Part model, mm, in its own coordinate system. Face numbers are marked on the shaded views. A direction names the side the tool comes from. Give positions to 0.01 mm unless a question says otherwise; leave off trailing zeros. Order: outer loops, then holes, each group sorted by start corner. A loop starts at its lowest first (then second) coordinate and runs counter-clockwise, first axis right, second up.
from build123d import *

# Parameters (mm, degrees)
SKETCH1_R                    = 37.5
BOSS_EXTRUDE1_DEPTH          = 6
CSK_FOR_M3_SFHCS1_AT_2_COUNT = 2
CSK_FOR_M3_SFHCS1_AT_2_PITCH = 17.32
CSK_FOR_M3_SFHCS1_AT_3_COUNT = 2
CSK_FOR_M3_SFHCS1_AT_3_PITCH = 17.32
SKETCH5_OUTSIDE_W            = 98.248
SKETCH5_OUTSIDE_H            = 98.248
SKETCH5_OUTSIDE_R            = 31
CUT_EXTRUDE2_DEPTH           = 3
F_4_0MM_DOWEL_HOLE1_D        = 4.2
F_4_0MM_DOWEL_HOLE1_DEPTH    = 10
F_4_0MM_DOWEL_HOLE1_TIP      = 1.2618073
CUT_EXTRUDE3_DEPTH           = 3.3
CHAMFER1_SIZE                = 0.5


with BuildPart() as part:
    # Sketch1 → Boss-Extrude1 (new body)
    with BuildSketch(Plane(origin=(0, 0, 0), x_dir=(1, 0, 0), z_dir=(0, 1, 0))):
        with Locations(Location((0, 0, 0), (0, 0, 270))):
            Circle(SKETCH1_R)
    extrude(amount=BOSS_EXTRUDE1_DEPTH)

    # Sketch3 → CSK for M3 SFHCS1 (revolve, cut)
    with BuildSketch(Plane(origin=(8.66, 6, 4.999853331), x_dir=(0, 0, 1), z_dir=(1, 0, 0))):
        Polygon((0, 0), (0, 11.021463052), (1.7, 10), (1.7, 2.66), (3.36, 1), (3.36, 0), align=None)
    csk_for_m3_sfhcs1 = revolve(axis=Axis((8.66, 12.35, 4.999853331), (0, -1, 0)), mode=Mode.SUBTRACT)

    # CSK for M3 SFHCS1 at 2: CSK for M3 SFHCS1 ×2
    with Locations(*[Vector(-0.5000000000000001, 0, -0.8660254037844387) * (i * CSK_FOR_M3_SFHCS1_AT_2_PITCH) for i in range(1, CSK_FOR_M3_SFHCS1_AT_2_COUNT)]):
        add(csk_for_m3_sfhcs1, mode=Mode.SUBTRACT)

    # CSK for M3 SFHCS1 at 3: CSK for M3 SFHCS1 ×2
    with Locations(*[(-i * CSK_FOR_M3_SFHCS1_AT_3_PITCH, 0, 0) for i in range(1, CSK_FOR_M3_SFHCS1_AT_3_COUNT)]):
        add(csk_for_m3_sfhcs1, mode=Mode.SUBTRACT)

    # Sketch5 outside → Cut-Extrude2 (cut)
    with BuildSketch(Plane(origin=(0, 6, 0), x_dir=(1, 0, 0), z_dir=(0, 1, 0))):
        Rectangle(SKETCH5_OUTSIDE_W, SKETCH5_OUTSIDE_H)
        with Locations(Location((0, 0, 0), (0, 0, 270))):
            Circle(SKETCH5_OUTSIDE_R, mode=Mode.SUBTRACT)
    extrude(amount=-CUT_EXTRUDE2_DEPTH, mode=Mode.SUBTRACT)

    # Ø4.0mm Dowel Hole1
    with Locations(Plane(origin=(0, 6, 0), x_dir=(1, 0, 0), z_dir=(0, 1, 0))):
        with Locations((17.67766953, 17.67766953), (-17.67766953, 17.67766953), (17.67766953, -17.67766953), (-17.67766953, -17.67766953)):
            Hole(F_4_0MM_DOWEL_HOLE1_D / 2, depth=F_4_0MM_DOWEL_HOLE1_DEPTH)
            with Locations((0, 0, -(F_4_0MM_DOWEL_HOLE1_DEPTH + F_4_0MM_DOWEL_HOLE1_TIP / 2))):  # 118° drill point
                Cone(0, F_4_0MM_DOWEL_HOLE1_D / 2, F_4_0MM_DOWEL_HOLE1_TIP, mode=Mode.SUBTRACT)

    # Sketch8 → Cut-Extrude3 (cut)
    with BuildSketch(Plane.XZ):
        Polygon((-14.22766953, 15.685811101), (-14.22766953, 19.669527958), (-17.67766953, 21.661386387), (-21.12766953, 19.669527958), (-21.12766953, 15.685811101), (-17.67766953, 13.693952672), align=None)
        Polygon((17.67766953, 13.693952672), (21.12766953, 15.685811101), (21.12766953, 19.669527958), (17.67766953, 21.661386387), (14.22766953, 19.669527958), (14.22766953, 15.685811101), align=None)
        Polygon((14.22766953, -19.669527958), (17.67766953, -21.661386387), (21.12766953, -19.669527958), (21.12766953, -15.685811101), (17.67766953, -13.693952672), (14.22766953, -15.685811101), align=None)
        Polygon((-14.22766953, -19.669527958), (-14.22766953, -15.685811101), (-17.67766953, -13.693952672), (-21.12766953, -15.685811101), (-21.12766953, -19.669527958), (-17.67766953, -21.661386387), align=None)
    extrude(amount=-CUT_EXTRUDE3_DEPTH, mode=Mode.SUBTRACT)

    # Chamfer1
    chamfer1_edges = [part.edges().sort_by_distance(p)[0] for p in [
        (15.95266953, 0, 14.689881887),
        (19.40266953, 0, 14.689881887),
        (21.12766953, 0, 17.67766953),
        (19.40266953, 0, 20.665457173),
        (15.95266953, 0, 20.665457173),
        (14.22766953, 0, 17.67766953),
        (-15.95266953, 0, 14.689881887),
        (-14.22766953, 0, 17.67766953),
        (-15.95266953, 0, 20.665457173),
        (-19.40266953, 0, 20.665457173),
        (-21.12766953, 0, 17.67766953),
        (-19.40266953, 0, 14.689881887),
        (-8.66, 0, 3.299853331),
        (-8.66, 6, 1.639853331),
        (0, 0, -37.5),
        (0, 0, -11.699706662),
        (0, 6, -13.359706662),
        (0, 3, -37.5),
        (0, 6, -31),
        (19.77766953, 6, -17.67766953),
        (-15.57766953, 6, 17.67766953),
        (19.77766953, 6, 17.67766953),
        (-15.57766953, 6, -17.67766953),
        (8.66, 0, 3.299853331),
        (8.66, 6, 1.639853331),
        (-15.95266953, 0, -20.665457173),
        (-14.22766953, 0, -17.67766953),
        (-15.95266953, 0, -14.689881887),
        (-19.40266953, 0, -14.689881887),
        (-21.12766953, 0, -17.67766953),
        (-19.40266953, 0, -20.665457173),
        (14.22766953, 0, -17.67766953),
        (15.95266953, 0, -20.665457173),
        (19.40266953, 0, -20.665457173),
        (21.12766953, 0, -17.67766953),
        (19.40266953, 0, -14.689881887),
        (15.95266953, 0, -14.689881887),
    ]]
    chamfer(chamfer1_edges, length=CHAMFER1_SIZE)


solid = part.part
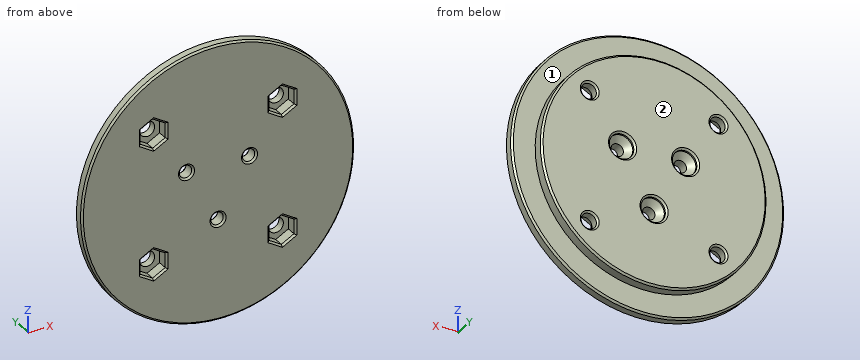
Item 1: Band-saw the part on A-A on x = 0. List the corners of the cut face in (y, z).
Item 2: Band-saw the part on B-B on z = 0. List the corners of the cut face in (x, y).
Item 3: Which spindle directions (+Z, -Z, +X, -X, +Y, -Y) get a long thin tool onto all of the face, cutting with end or side? Do the marked faces 1 and 2. Say none if no direction does.
Item 4: Drill centre lines: probe 1 along X at (y, z) = (5, 5); probe 2 along Z at (x, y) = (0, 2.1); probe 3 along X at (y, z) = (2, 16.5). Where is each one in solid material? Low to high.
Item 5: Drop flat-ended pins along their axis: P1, Ø5.5, axis at x = 17.68, z = 17.68, coming from the -Y side; P2, Ø3, axis at x = 8.66, z = 5, coming from the -Y side; P3, Ø5.5, axis at x = -8.66, z = 5, coming from the +Y side; P4, Ø3, axis at x = 29, y = 5.5, coming from the +Z side. Give the stop position or say it passes through.
Working result:
1. outline: (0, -37) - (0.5, -37.5) - (2.5, -37.5) - (3, -37) - (3, -31) - (5.5, -31) - (6, -30.5) - (6, -13.86) - (5.5, -13.36) - (5, -13.36) - (3.34, -11.7) - (0.5, -11.7) - (0, -12.2) - close; (0, -7.8) - (0.5, -8.3) - (3.34, -8.3) - (5, -6.64) - (5.5, -6.64) - (6, -6.14) - (6, 30.5) - (5.5, 31) - (3, 31) - (3, 37) - (2.5, 37.5) - (0.5, 37.5) - (0, 37) - close
2. outline: (-37.5, 0.5) - (-37, 0) - (37, 0) - (37.5, 0.5) - (37.5, 2.5) - (37, 3) - (31, 3) - (31, 5.5) - (30.5, 6) - (-30.5, 6) - (-31, 5.5) - (-31, 3) - (-37, 3) - (-37.5, 2.5) - close
3. face 1: +Y
3. face 2: +Z, -Z, +X, -X, +Y
4. probe 1: x = -30.59 to -12.02, -5.3 to 5.3, 12.02 to 30.59
4. probe 2: z = -37.5 to -11.7, -8.3 to 37.5
4. probe 3: x = -33.67 to -21.13, -14.23 to 14.23, 21.13 to 33.67
5. P1: stops at y = 3.3
5. P2: passes through
5. P3: stops at y = 4.39
5. P4: stops at z = 14.31
